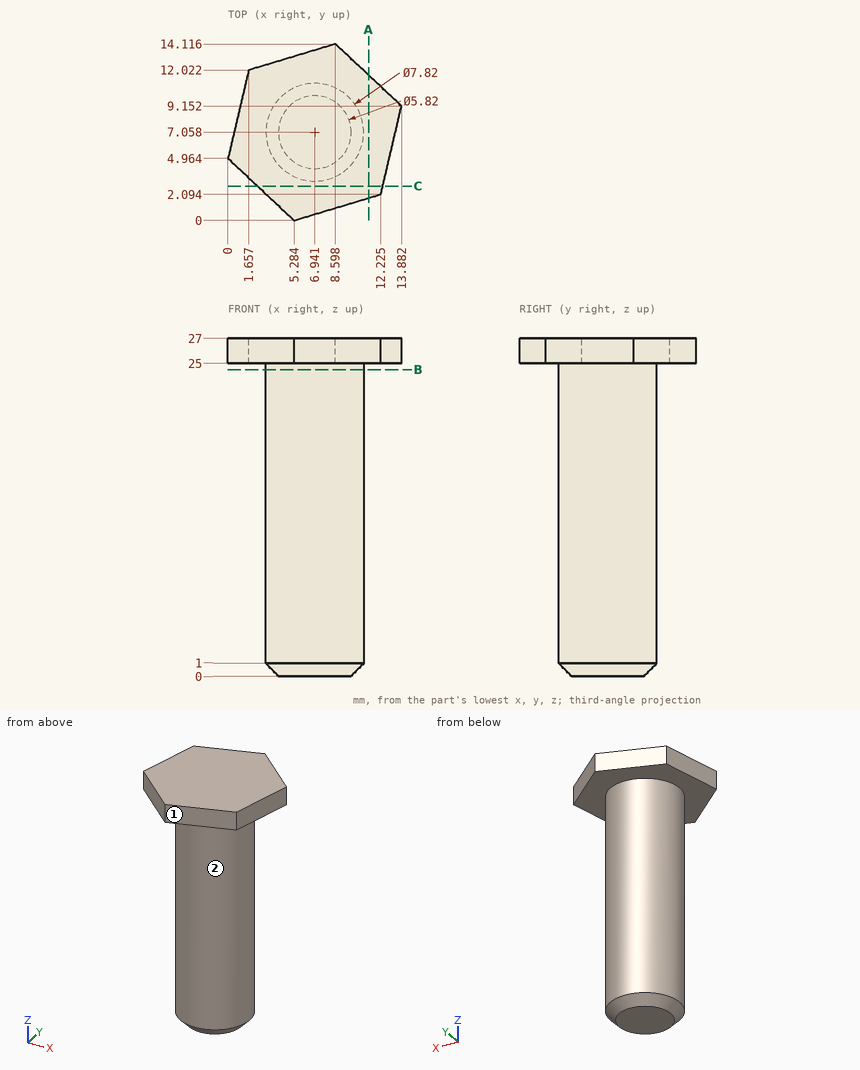
Verification items for this drawing (mm, ordinates from the low corner). A direction names the side the tool comes from. Round coordinates to 2 decimals unless told otherwise and drop trailing zeros. Order: outer loops, then holes, each group sorted by start corner. A loop starts at its lowest first (then second) coordinate and runs counter-clockwise, first axis right, second up. Notation, with made-up numbers: (-25.75, -8) - (9.25, -8) arc R15 ccw to (9.25, 13) - close; hole circle Ø10 at (-24, 84). An arc over 180 degrees is marked (long way). Use CSV: the item, a comma, the result in double quotes.
(1) Section check C-C on y = 2.75. Record the boundary of the cut face in (x, z).
Entries:
outline,"(2.36, 25) - (12.38, 25) - (12.38, 27) - (2.36, 27) - close"
(2) Access from +Z, -Z, +X, -X, +Y, -Y to the whole of each face (thin tool, end or side, straight path). Record for the marked faces 1 and 2.
Entries:
face 1,"+Z, -Z, +X, -Y"
face 2,"-Z"
(3) Section check B-B on z = 24.5. Record the boundary of the cut face in (x, y), and give its area (3 significant figures).
Entries:
outline,"circle Ø7.82 at (6.94, 7.06)"
area,"48.0 mm^2"
(4) Section check A-A on x = 11.25. Record the boundary of the cut face in (y, z) (1 decimal).
Entries:
outline,"(1.8, 25) - (11.6, 25) - (11.6, 27) - (1.8, 27) - close"
(5) Gauge pin test, flat ends, axial feed: pin 1 Ø5 at (y, z) = (6, 19.5) entering from -X; pin 2 Ø4 at (x, y) = (10, 8) entering from -Z; pin 3 Ø1 at (y, z) = (3.5, 22) entering from -X (1 decimal); pin 4 Ø6 at (y, z) = (3, 7.5) entering from +X (1 decimal). Record the tip position at first contact, or that the pin passes through.
Entries:
pin 1,"x = 3.03"
pin 2,"z = 0"
pin 3,"x = 4.5"
pin 4,"x = 10.7"
(6) Thickness scan on probe 1 along Z at (x, y) = (6.25, 12.75); probe 2 along X at (y, z) = (4, 15.25) (1 decimal); probe 3 along Z at (x, y) = (4, 7.5) (1 decimal). Record the ranges inside material, lowest first. Write a range as from..to.
Entries:
probe 1,"25..27"
probe 2,"4.5..9.4"
probe 3,"0.1..27"
